Read the model definition and answer for the solid it produces. Units are mm, in the model's axes. A direction names the side the tool comes from. Give positions to 0.01 mm unless a question says otherwise; leave off trailing zeros. Loops run counter-clockwise (first coordinate to the right, second up) from the corner with the lowest first, then second, coordinate; pieces in that order, holes last.
(1) Which of the six approach directions +Z, -Z, +X, -X, +Y, -Y give full straight-line access (tool end or side, diameter ignored) to faces 4 (the face through (-3.84, -1.216, 1.115)), 5 (the face through (-3.175, 0, 3)), 6 (the face through (-3.175, 0, -3)), 7 (the face through (1.49, 0.03, 0.47))?
(2) Find section A-A, the plane x = -1.75. Write down the section's boundary in (y, z) (3 decimals).
(3) Straight lines are drawn through the part: probe 1 along X at (y, z) = (-1.35, 0) (1 decimal); probe 2 along Y at (x, z) = (-5, 1.25); probe 3 along Y at (x, z) = (-2.5, 0.5). For each, find the intervals that lie inside material, in ascending order.
(4) Find section D-D, the plane x = 0.5. Write down the section's boundary in (y, z), then the cut area to 3 significant figures.
(5) Each of these flat-tipped pins is pushed along its axis until it touches: P1, Ø2, axis at x = -4.5, y = -1.5, coming from the +Z side; P2, Ø2, axis at y = -0.5, z = 0, coming from the -X side; P3, Ø2.5, axis at y = 0, z = 0, coming from the -X side. Where does it stop, or does it pass through?
(6) Determine the mould class of faces 1 (the face through (-1.155, -0.02, 1.284)), 2 (the face through (-6.375, 2, 0)), 3 (the face through (-4.753, 1.865, -1.43)) for opening direction Z: pulls with the +Z half, pulls with the -Z half, needs draft (parallel to the pull), parting line crosses it, or undercut.
(7) Find section B-B, the plane z = -0.5. Write down the section's boundary in (x, y) (3 decimals).
```python
from build123d import *

# Parameters (mm, degrees)
F0_R     = 1.5625
F1_DEPTH = 2.35
F3_DEPTH = 3.2
F5_D     = 3.3
F5_DEPTH = 5
F5_TIP   = 0.9914200214


with BuildPart() as f1:
    # F0 (on Front) → F1 (new body, symmetric)
    with BuildSketch(Plane.XZ):
        with BuildLine():
            Line((0, 3.175), (-3.175, 3.175))
            Line((-3.175, 3.175), (-3.175, -3.175))
            Line((-3.175, -3.175), (0, -3.175))
            ThreePointArc((0, -3.175), (3.175, 0), (0, 3.175))
        make_face()
        Circle(F0_R, mode=Mode.SUBTRACT)
    extrude(amount=F1_DEPTH, both=True)

    # F2 (on face) → F3 (join)
    with BuildSketch(Plane(origin=(-3.175, 0, 0), x_dir=(0, -1, 0), z_dir=(-1, 0, 0))):
        with BuildLine():
            ThreePointArc((-2.35, 0), (0, -2.35), (2.35, 0))
            ThreePointArc((2.35, 0), (0, 2.35), (-2.35, 0))
        make_face()
    extrude(amount=F3_DEPTH)

    # F5
    with Locations(Plane(origin=(-6.375, 0, 0), x_dir=(0, -1, 0), z_dir=(-1, 0, 0))):
        with Locations((0, 0)):
            Hole(F5_D / 2, depth=F5_DEPTH)
            with Locations((0, 0, -(F5_DEPTH + F5_TIP / 2))):  # 118° drill point
                Cone(0, F5_D / 2, F5_TIP, mode=Mode.SUBTRACT)


solid = f1.part
```
Entries:
1. face 4: -X
1. face 5: +Z, -X
1. face 6: -Z, -X
1. face 7: +Y, -Y
2. outline: (-2.35, -3.175) - (2.35, -3.175) - (2.35, 3.175) - (-2.35, 3.175) - close; hole circle Ø3.3 at (0, 0)
3. probe 1: x = 1.6 to 3.2
3. probe 2: y = -1.99 to -1.08, 1.08 to 1.99
3. probe 3: y = -2.35 to -1.57, 1.57 to 2.35
4. outline: (-2.35, -3.14) - (2.35, -3.14) - (2.35, -1.48) - (-2.35, -1.48) - close; (-2.35, 1.48) - (2.35, 1.48) - (2.35, 3.14) - (-2.35, 3.14) - close
4. area: 15.6 mm2
5. P1: stops at z = 2.3
5. P2: stops at x = 1.2
5. P3: stops at x = -1.13
6. face 1: undercut
6. face 2: needs draft
6. face 3: parting line crosses it
7. outline: (-6.375, -2.296) - (-3.175, -2.296) - (-3.175, -2.35) - (-1.48, -2.35) - (-1.48, -1.572) - (-6.375, -1.572) - close; (-6.375, 1.572) - (-1.48, 1.572) - (-1.48, 2.35) - (-3.175, 2.35) - (-3.175, 2.296) - (-6.375, 2.296) - close; (1.48, -2.35) - (3.135, -2.35) - (3.135, 2.35) - (1.48, 2.35) - close
